The model under review builds one solid part; all positions refer to its coordinate system, in mm. Face numbers are marked on the shaded views. A direction names the side the tool comes from. Give positions to 0.01 mm unless a question says otherwise; leave off trailing zeros. Loops run counter-clockwise (first coordinate to the right, second up) from the corner with the lowest first, then second, coordinate; pieces in that order, holes last. Notation, with made-up numbers: M 37.5,-36 L 53.5,-36 A12 cw 53.5,-20 Z; hole C 0.5,73.5 d10. An arc over 180 degrees is marked long. Return JSON: item names as keys, results as strings.
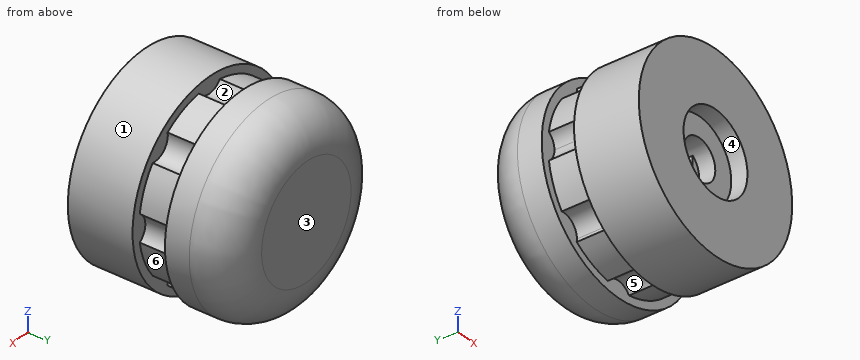
```python
from build123d import *

# Parameters (mm, degrees)
SALIENTE_EXTRUIR3_DEPTH = 20
CROQUIS13_R             = 12
SALIENTE_EXTRUIR4_DEPTH = 8
SALIENTE_EXTRUIR5_START = -8
CROQUIS15_R             = 12
SALIENTE_EXTRUIR5_DEPTH = 8
CROQUIS16_R             = 5
CORTAR_EXTRUIR6_DEPTH   = 2
CROQUIS17_R             = 2.5
CORTAR_EXTRUIR7_DEPTH   = 2
CORTAR_EXTRUIR8_DEPTH   = 7
REDONDEO2_R             = 5


with BuildPart() as part:
    # Croquis12 → Saliente-Extruir3 (new body)
    with BuildSketch(Plane(origin=(0, 0, 0), x_dir=(1, 0, 0), z_dir=(0, 1, 0))):
        with BuildLine():
            ThreePointArc((10.875, -1.653594569), (10, 0), (10.875, 1.653594569))
            ThreePointArc((10.875, 1.653594569), (10.162674858, 4.209517756), (8.859054179, 6.520518312))
            ThreePointArc((8.859054179, 6.520518312), (7.071067812, 7.071067812), (6.520518312, 8.859054179))
            ThreePointArc((6.520518312, 8.859054179), (4.209517756, 10.162674858), (1.653594569, 10.875))
            ThreePointArc((1.653594569, 10.875), (0, 10), (-1.653594569, 10.875))
            ThreePointArc((-1.653594569, 10.875), (-4.209517756, 10.162674858), (-6.520518312, 8.859054179))
            ThreePointArc((-6.520518312, 8.859054179), (-6.494110095, 8.672996418), (-6.485281374, 8.485281374))
            ThreePointArc((-6.485281374, 8.485281374), (-7.210045241, 6.94457608), (-8.859054179, 6.520518312))
            ThreePointArc((-8.859054179, 6.520518312), (-10.162674858, 4.209517756), (-10.875, 1.653594569))
            ThreePointArc((-10.875, 1.653594569), (-10.232233047, 0.935414347), (-10, 0))
            ThreePointArc((-10, 0), (-10.232233047, -0.935414347), (-10.875, -1.653594569))
            ThreePointArc((-10.875, -1.653594569), (-10.162674858, -4.209517756), (-8.859054179, -6.520518312))
            ThreePointArc((-8.859054179, -6.520518312), (-7.210045241, -6.94457608), (-6.485281374, -8.485281374))
            ThreePointArc((-6.485281374, -8.485281374), (-6.494110095, -8.672996418), (-6.520518312, -8.859054179))
            ThreePointArc((-6.520518312, -8.859054179), (-4.209517756, -10.162674858), (-1.653594569, -10.875))
            ThreePointArc((-1.653594569, -10.875), (0, -10), (1.653594569, -10.875))
            ThreePointArc((1.653594569, -10.875), (4.209517756, -10.162674858), (6.520518312, -8.859054179))
            ThreePointArc((6.520518312, -8.859054179), (7.071067812, -7.071067812), (8.859054179, -6.520518312))
            ThreePointArc((8.859054179, -6.520518312), (10.162674858, -4.209517756), (10.875, -1.653594569))
        make_face()
    extrude(amount=SALIENTE_EXTRUIR3_DEPTH)

    # Croquis13 → Saliente-Extruir4 (add)
    with BuildSketch(Plane.XZ):
        with Locations(Location((0, 0, 0), (0, 0, 270))):
            Circle(CROQUIS13_R)
    extrude(amount=-SALIENTE_EXTRUIR4_DEPTH)

    # Croquis15 → Saliente-Extruir5 (add)
    with BuildSketch(Plane(origin=(0, 20, 0), x_dir=(1, 0, 0), z_dir=(0, 1, 0)).offset(SALIENTE_EXTRUIR5_START)):
        with Locations(Location((0, 0, 0), (0, 0, 90))):
            Circle(CROQUIS15_R)
    extrude(amount=SALIENTE_EXTRUIR5_DEPTH)

    # Croquis16 → Cortar-Extruir6 (cut)
    with BuildSketch(Plane.XZ):
        with Locations(Location((0, 0, 0), (0, 0, 270))):
            Circle(CROQUIS16_R)
    extrude(amount=-CORTAR_EXTRUIR6_DEPTH, mode=Mode.SUBTRACT)

    # Croquis17 → Cortar-Extruir7 (cut)
    with BuildSketch(Plane.XZ.offset(-2)):
        with Locations(Location((0, 0, 0), (0, 0, 270))):
            Circle(CROQUIS17_R)
    extrude(amount=-CORTAR_EXTRUIR7_DEPTH, mode=Mode.SUBTRACT)

    # Croquis18 → Cortar-Extruir8 (cut)
    with BuildSketch(Plane.XZ.offset(-4)):
        with BuildLine():
            Line((-1.5, 2), (-1.5, -2))
            ThreePointArc((-1.5, -2), (0, -2.5), (1.5, -2))
            Line((1.5, -2), (1.5, 2))
            ThreePointArc((1.5, 2), (0, 2.5), (-1.5, 2))
        make_face()
    extrude(amount=-CORTAR_EXTRUIR8_DEPTH, mode=Mode.SUBTRACT)

    # Redondeo2
    redondeo2_edges = [part.edges().sort_by_distance(p)[0] for p in [
        (0, 20, 12),
    ]]
    fillet(redondeo2_edges, radius=REDONDEO2_R)


solid = part.part
```
1) Consider section B-B on y = 1.25. Write out the cut boundary in (x, z).
From the geometry:
{"outline": "C 0,0 d24; hole C 0,0 d10"}
2) Tool access review of the marked faces 4, 5 and 6: name each direction out of +Z, -Z, +X, -X, +Y, -Y from which nothing blocks a thin tool from reaching the whole face with its end or side.
From the geometry:
{"face 4": "-Y", "face 5": "-Z", "face 6": "-Z, +X"}
3) Consider section C-C on y = 16.5. Write out the cut boundary in (x, z), then the cut area to 3 significant figures.
From the geometry:
{"outline": "C 0,0 d23.54", "area": "435 mm²"}
4) Insertion check: pin 1 (2 mm diameter, centred on y = 10.5, z = -1, fed in from +X) (3 decimals); pin 2 (6 mm diameter, centred on y = 14.5, z = 6, fed in from +X); pin 3 (1.5 mm diameter, centred on x = 1, y = 3, fed in from -Z). Each pin has a flat end and moves straight along its axis. Give the tip position at first contact, or say it passes through.
From the geometry:
{"pin 1": "x = 10.875", "pin 2": "x = 11.62", "pin 3": "z = -12"}
5) The part is to be moulded in two halves that separate along Y. For the marked faces 1, 2 and 3, say which applies: released by +Y, released by -Y, zero draft, split by the parting line, or undercut.
From the geometry:
{"face 1": "zero draft", "face 2": "undercut", "face 3": "released by +Y"}
6) Consider section A-A on y = 9.25. Write out the cut boundary in (x, z) (3 decimals).
From the geometry:
{"outline": "M -10.875,-1.654 A11 ccw -8.859,-6.521 A2 cw -6.521,-8.859 A11 ccw -1.654,-10.875 A2 cw 1.654,-10.875 A11 ccw 6.521,-8.859 A2 cw 8.859,-6.521 A11 ccw 10.875,-1.654 A2 cw 10.875,1.654 A11 ccw 8.859,6.521 A2 cw 6.521,8.859 A11 ccw 1.654,10.875 A2 cw -1.654,10.875 A11 ccw -6.521,8.859 A2 cw -8.859,6.521 A11 ccw -10.875,1.654 A2 cw Z; hole M -1.5,-2 A2.5 ccw 1.5,-2 L 1.5,2 A2.5 ccw -1.5,2 Z"}
7) Wall thickness on L1, parallel to X at y = 0.55, z = 0; L2, parallel to X at y = 7.5, z = 0; L3, parallel to Z at x = 0, y = 9: over which ranges is each line inside the solid? List them lowest first. Write a range as from..to.
From the geometry:
{"L1": "-12..-5, 5..12", "L2": "-12..-1.5, 1.5..12", "L3": "-10..-2.5, 2.5..10"}
